Check sheet for the drawn part. Datum: minimum x, y, z corner. Units: mm. Coordinates: 2 decimals unless noted, no trailing zeros. Order: outer loops, then holes, each group sorted by start corner. A loop starts at its lowest first (then second) coordinate and runs counter-clockwise, first axis right, second up. Notation, with made-up numbers: (71, 8) -> (101, 8) arc R16 ccw to (101, 14) -> close; hole circle Ø1 at (66, 69). An arc over 180 degrees is marked (long way). Write item = value, one per line. Start each with the question number.
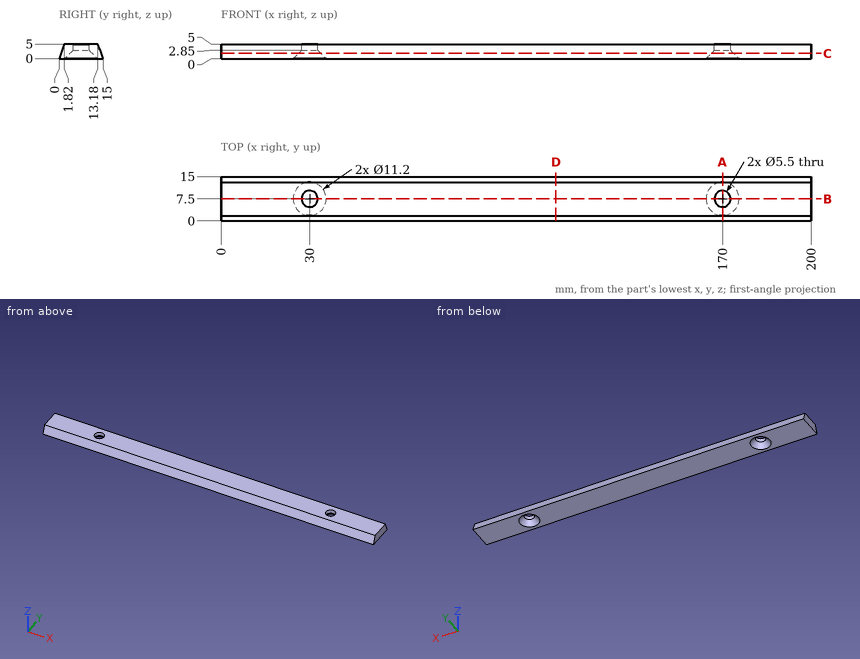
Item 1: Gauge pin test, flat ends, axial feed: P1, Ø6.5, axis at x = 30, y = 7.5, coming from the -Z side; P2, Ø2, axis at x = 38.5, z = 1.5, coming from the -Y side. Record the tip position at first contact, or that the pin passes through.
Item 2: Section check C-C (z = 1.8). Record the boundary of the cut face in (x, y) (3 decimals), then the cut area to 3 significant figures.
Item 3: Section check D-D (x = 113.5). Record the boundary of the cut face in (y, z), then the cut area to 3 significant figures.
Item 4: Section check A-A (x = 170). Record the boundary of the cut face in (y, z).
Item 5: Section check B-B (y = 7.5). Record the boundary of the cut face in (x, z), then the cut area to 3 significant figures.
Item 6: Thickness scan on line 1 (X direction, y = 7.25, z = 3); line 2 (X direction, y = 9.75, z = 2.6) (1 decimal); line 3 (Y direction, x = 30, z = 4.35). Record the ranges inside material, lowest first.
Filled sheet:
q1.P1 = 2.35
q1.P2 = 0.18
q2.outline = (0, 0.655) -> (200, 0.655) -> (200, 14.345) -> (0, 14.345) -> close; hole circle Ø7.6 at (30, 7.5); hole circle Ø7.6 at (170, 7.5)
q2.area = 2,650 mm^2
q3.outline = (0, 0) -> (15, 0) -> (13.18, 5) -> (1.82, 5) -> close
q3.area = 65.9 mm^2
q4.outline = (0, 0) -> (1.9, 0) -> (4.75, 2.85) -> (4.75, 5) -> (1.82, 5) -> close; (10.25, 2.85) -> (13.1, 0) -> (15, 0) -> (13.18, 5) -> (10.25, 5) -> close
q5.outline = (0, 0) -> (24.4, 0) -> (27.25, 2.85) -> (27.25, 5) -> (0, 5) -> close; (32.75, 2.85) -> (35.6, 0) -> (164.4, 0) -> (167.25, 2.85) -> (167.25, 5) -> (32.75, 5) -> close; (172.75, 2.85) -> (175.6, 0) -> (200, 0) -> (200, 5) -> (172.75, 5) -> close
q5.area = 929 mm^2
q6.line_1 = 0 to 27.26, 32.74 to 167.26, 172.74 to 200
q6.line_2 = 0 to 28, 32 to 168, 172 to 200
q6.line_3 = 1.58 to 4.75, 10.25 to 13.42
